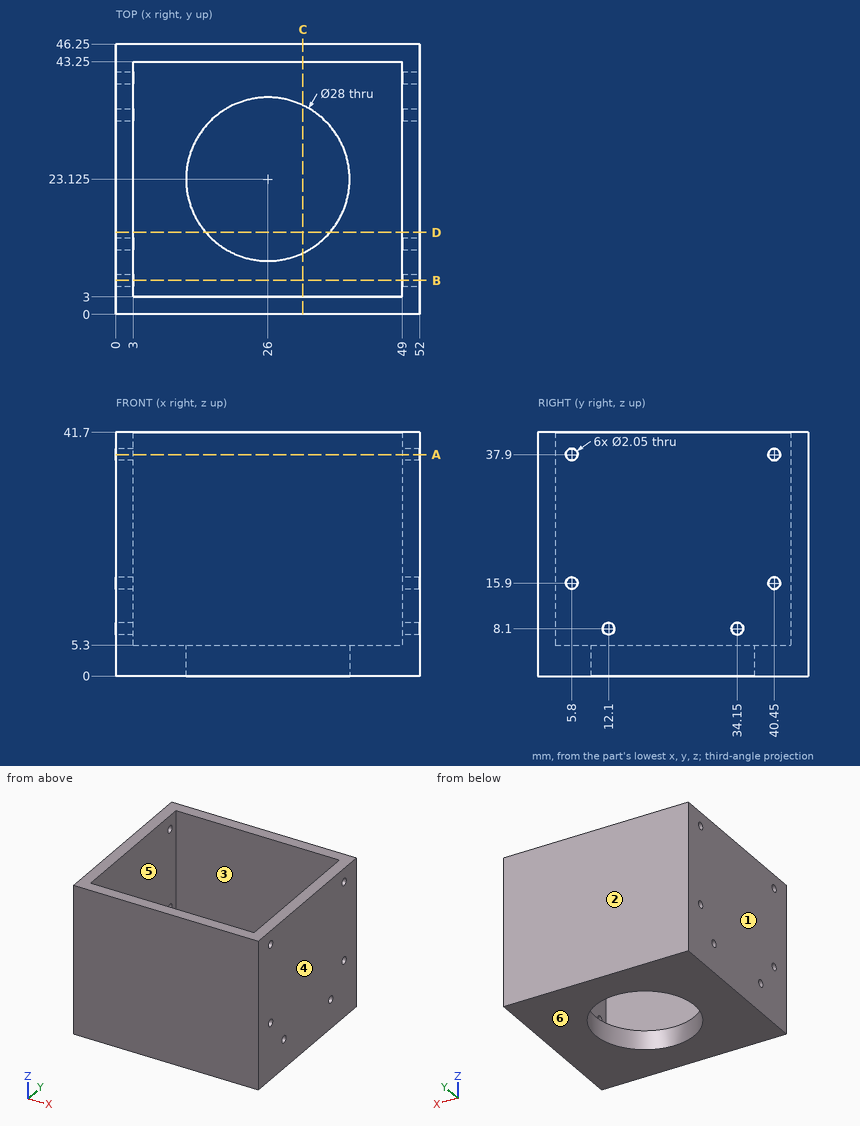
The figure shows three views and two pictorial views of one solid part (mm, origin at its lowest corner). Answer the questions. A direction names the side the tool comes from. Give positions to 0.01 mm unless a question says otherwise; leave off trailing zeros. Order: outer loops, then holes, each group sorted by start corner. A loop starts at its lowest first (then second) coordinate and runs counter-clockwise, first axis right, second up. Notation, with made-up numbers: (6.5, 88.5) -> (61.5, 88.5) arc R26 cw to (61.5, 113.5) -> close; hole circle Ø7 at (-2, 89.25). An arc over 180 degrees is marked (long way). One line per item, written item: value.
1) Find section A-A, the plane z = 37.9. Determine the outline of the cut face in (x, y) (3 decimals).
Reported:
outline: (0, 0) -> (52, 0) -> (52, 4.775) -> (49, 4.775) -> (49, 3) -> (3, 3) -> (3, 4.775) -> (0, 4.775) -> close; (0, 6.825) -> (3, 6.825) -> (3, 39.425) -> (0, 39.425) -> close; (0, 41.475) -> (3, 41.475) -> (3, 43.25) -> (49, 43.25) -> (49, 41.475) -> (52, 41.475) -> (52, 46.25) -> (0, 46.25) -> close; (49, 6.825) -> (52, 6.825) -> (52, 39.425) -> (49, 39.425) -> close
2) Find section C-C, the plane x = 32. Determine the outline of the cut face in (y, z), plus the area to 3 significant figures.
Reported:
outline: (0, 0) -> (10.48, 0) -> (10.48, 5.3) -> (3, 5.3) -> (3, 41.7) -> (0, 41.7) -> close; (35.77, 0) -> (46.25, 0) -> (46.25, 41.7) -> (43.25, 41.7) -> (43.25, 5.3) -> (35.77, 5.3) -> close
area: 329 mm^2
3) Flat-ended cylindrical pins translate along their axes: P1, Ø1.8, axis at y = 5.8, z = 15.9, coming from the -X side; P2, Ø10, axis at x = 15.5, y = 38, coming from the +Z side; P3, Ø8, axis at y = 5.5, z = 7.5, coming from the -X side. Find the tip coordinate at first contact, or state that the pin passes through.
Reported:
P1: passes through
P2: stops at z = 5.3
P3: stops at x = 0
4) Determine the mould class of the marked faces 1, 2, 3 and 4 for opening direction X: pulls with the +X half, pulls with the -X half, needs draft (parallel to the pull), parting line crosses it, or undercut.
Reported:
face 1: pulls with the -X half
face 2: needs draft
face 3: undercut
face 4: pulls with the +X half
5) Find section D-D, the plane y = 14. Determine the outline of the cut face in (x, z).
Reported:
outline: (0, 0) -> (15.38, 0) -> (15.38, 5.3) -> (3, 5.3) -> (3, 41.7) -> (0, 41.7) -> close; (36.62, 0) -> (52, 0) -> (52, 41.7) -> (49, 41.7) -> (49, 5.3) -> (36.62, 5.3) -> close
6) A tool of negligible diameter and unlimited length cuts with its end or side. For the marked faces 5 and 6, from which of +Z, -Z, +X, -X, +Y, -Y can it reach the whole face along a straight path? Write none if from no direction.
Reported:
face 5: +Z
face 6: -Z, +X, -X, +Y, -Y
7) Find the intervals of material crossed by line 1 (Z direction, x = 2.1, y = 40.45) (3 decimals); line 2 (Y direction, x = 1, z = 8); line 3 (Y direction, x = 50.7, z = 15.9) (3 decimals), in increasing order.
Reported:
line 1: z = 0 to 14.875, 16.925 to 36.875, 38.925 to 41.7
line 2: y = 0 to 11.08, 13.12 to 33.13, 35.17 to 46.25
line 3: y = 0 to 4.775, 6.825 to 39.425, 41.475 to 46.25
8) Find section B-B, the plane y = 5.8. Determine the outline of the cut face in (x, z) (3 decimals), plus the area to 3 significant figures.
Reported:
outline: (0, 0) -> (52, 0) -> (52, 14.875) -> (49, 14.875) -> (49, 5.3) -> (3, 5.3) -> (3, 14.875) -> (0, 14.875) -> close; (0, 16.925) -> (3, 16.925) -> (3, 36.875) -> (0, 36.875) -> close; (0, 38.925) -> (3, 38.925) -> (3, 41.7) -> (0, 41.7) -> close; (49, 16.925) -> (52, 16.925) -> (52, 36.875) -> (49, 36.875) -> close; (49, 38.925) -> (52, 38.925) -> (52, 41.7) -> (49, 41.7) -> close
area: 469 mm^2
